Geometry check sheet. Reference: drawing and pictorial views, mm from the part's lowest x, y, z. A direction names the side the tool comes from. Round coordinates to 2 decimals unless told otherwise and drop trailing zeros. Order: outer loops, then holes, each group sorted by start corner. A loop starts at its lowest first (then second) coordinate and runs counter-clockwise, first axis right, second up. Notation, with made-up numbers: (86.5, 76) -> (109.5, 76) arc R12 cw to (109.5, 90) -> close; hole circle Ø6 at (13.5, -31). An arc over 180 degrees is marked (long way). Return JSON: item names as keys, results as strings. Group by question number.
1) Depth check by flat-ended pin: pin 1 (7.5 mm diameter, centred on y = 11.5, z = 17, fed in from +X); pin 2 (3 mm diameter, centred on y = 12.7, z = 10.16, fed in from -X) (3 decimals); pin 3 (12.5 mm diameter, centred on y = 8.5, z = 27, fed in from -X); pin 4 (12.5 mm diameter, centred on x = 15, z = 20, fed in from -Y). Enter the tip coordinate at first touch or a pass-through.
2) Section check D-D on z = 21. Enter the section's corners in (x, y), plus the area to 3 significant figures.
3) Section check C-C on x = 35. Enter the section's corners in (y, z).
4) Tool access check on the marked faces 4, 5, 6 and 7. Record the directions out of +Z, -Z, +X, -X, +Y, -Y that give a thin tool (end or side, any length) a straight path to the whole face; none if there is none.
5) Section check A-A on z = 26.67. Enter the section's corners in (x, y) (3 decimals).
6) Scan lines: L1, parallel to Y at x = 27, z = 10; L2, parallel to Y at x = 31.5, z = 4.5; L3, parallel to X at y = 51.5, z = 28.5. Record each from-to range of solid material in increasing order.
7) Draft check along Y on the marked faces 1, 2 and 3. Enter one of: pulls with the +Y half, pulls with the -Y half, needs draft (parallel to the pull), parting line crosses it, or undercut.
8) Section check B-B on y = 12.7. Enter the section's corners in (x, z) (3 decimals).
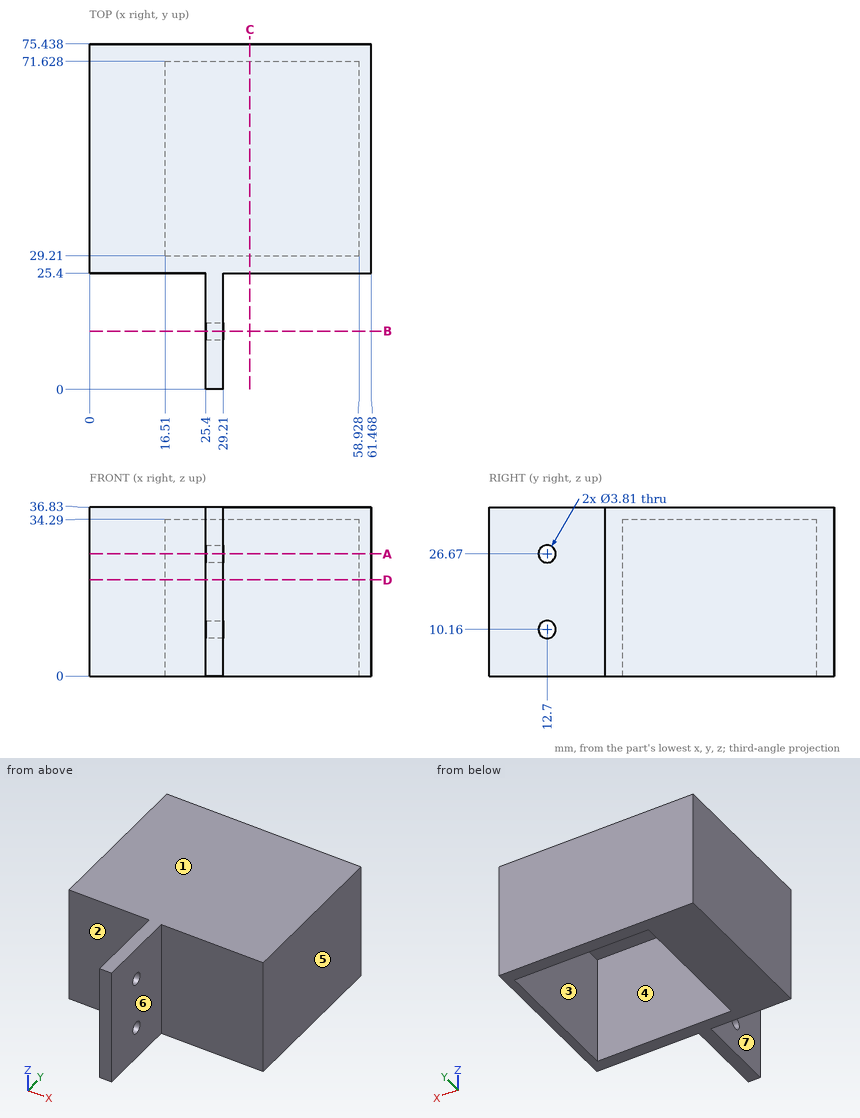
Check result:
{
 "1": {"pin 1": "x = 29.21", "pin 2": "through", "pin 3": "x = 25.4", "pin 4": "y = 25.4"},
 "2": {"outline": "(0, 25.4) -> (25.4, 25.4) -> (25.4, 0) -> (29.21, 0) -> (29.21, 25.4) -> (61.47, 25.4) -> (61.47, 75.44) -> (0, 75.44) -> close; hole (16.51, 29.21) -> (58.93, 29.21) -> (58.93, 71.63) -> (16.51, 71.63) -> close", "area": "1,370 mm^2"},
 "3": {"outline": "(25.4, 0) -> (29.21, 0) -> (29.21, 34.29) -> (71.63, 34.29) -> (71.63, 0) -> (75.44, 0) -> (75.44, 36.83) -> (25.4, 36.83) -> close"},
 "4": {"face 4": "-Z", "face 5": "+Z, -Z, +X, +Y, -Y", "face 6": "+Z, -Z, +X, -Y", "face 7": "+Z, -Z, -X, -Y"},
 "5": {"outline": "(0, 25.4) -> (25.4, 25.4) -> (25.4, 14.605) -> (29.21, 14.605) -> (29.21, 25.4) -> (61.468, 25.4) -> (61.468, 75.438) -> (0, 75.438) -> close; (25.4, 0) -> (29.21, 0) -> (29.21, 10.795) -> (25.4, 10.795) -> close; hole (16.51, 29.21) -> (58.928, 29.21) -> (58.928, 71.628) -> (16.51, 71.628) -> close"},
 "6": {"L1": "0 to 10.8, 14.6 to 29.21, 71.63 to 75.44", "L2": "25.4 to 29.21, 71.63 to 75.44", "L3": "0 to 16.51, 58.93 to 61.47"},
 "7": {"face 1": "needs draft", "face 2": "pulls with the -Y half", "face 3": "undercut"},
 "8": {"outline": "(25.4, 0) -> (29.21, 0) -> (29.21, 8.255) -> (25.4, 8.255) -> close; (25.4, 12.065) -> (29.21, 12.065) -> (29.21, 24.765) -> (25.4, 24.765) -> close; (25.4, 28.575) -> (29.21, 28.575) -> (29.21, 36.83) -> (25.4, 36.83) -> close"}
}
